Model file for the job. Use its own axes, mm. Coordinates: 2 decimals unless noted, no trailing zeros. Loops run counter-clockwise (first coordinate to the right, second up) from the corner with the lowest first, then second, coordinate; pieces in that order, holes last. Notation, with made-up numbers: (-27.75, 61) - (26.25, 61) arc R26 ccw to (26.25, 99) - close; hole circle Ø6 at (-31, -19). An arc over 180 degrees is marked (long way). Write each question's results on one line, items separated by ' | '. Start each with the question number.
```python
from build123d import *

# Parameters (mm, degrees)
EXTRUDE_1_DEPTH = 7
FILLET_1_R      = 10


with BuildPart() as part:
    # 草图1 → 凸台-拉伸1 (new body)
    with BuildSketch(Plane.XY):
        Polygon((-79.488423121, 60.813672833), (-61.488423121, 60.813672833), (-35.816291974, -24.186327167), (-51.816291974, -24.186327167), (-51.816291974, -40.186327167), (-16.816291974, -40.186327167), (-16.816291974, 60.813672833), (40.511576879, 60.813672833), (40.511576879, 40.813672833), (10.511576879, -55.186327167), (-79.488423121, -55.186327167), align=None)
    extrude(amount=EXTRUDE_1_DEPTH)

    # 圆角1
    fillet_1_edges = [part.edges().sort_by_distance(p)[0] for p in [
        (40.511576879, 40.813672833, 3.5),
    ]]
    fillet(fillet_1_edges, radius=FILLET_1_R)


solid = part.part
```
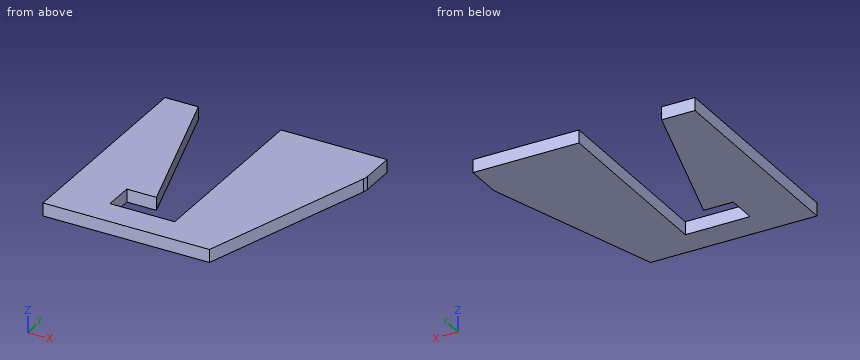
Q1. Pin check, flat tips, straight feed: pin 1 (4 mm diameter, centred on y = -10, z = 3.5, fed in from +X); pin 2 (3.5 mm diameter, centred on y = -29.5, z = 4.5, fed in from +X). Stop position of each tip, or through.
Q2. Drill centre lines: L1, parallel to X at y = -14.5, z = 4.75; L2, parallel to X at y = 15, z = 4.75; L3, parallel to Y at x = -25, z = 4.25. Where is each one in solid material? Low to high. Write a range as from..to.
Q3. Cut at A-A (x = -39). List the corners of the cut face in (y, z), and give its area (3 significant figures).
Q4. Cut at B-B (y = -18). List the corners of the cut face in (x, z).
Q5. Cut at D-D (x = 17.5). List the corners of the cut face in (y, z).
Q6. Cut at C-C (z = 1.5). List the corners of the cut face in (x, y).
Check result:
1) pin 1: x = 25.26 | pin 2: x = 19.09
2) L1: -79.49..-38.74, -16.82..23.23 | L2: -79.49..-47.65, -16.82..32.44 | L3: -55.19..-40.19
3) outline: (-55.19, 0) - (-40.19, 0) - (-40.19, 7) - (-55.19, 7) - close; (-24.19, 0) - (-13.65, 0) - (-13.65, 7) - (-24.19, 7) - close | area: 179 mm²
4) outline: (-79.49, 0) - (-37.68, 0) - (-37.68, 7) - (-79.49, 7) - close; (-16.82, 0) - (22.13, 0) - (22.13, 7) - (-16.82, 7) - close
5) outline: (-32.82, 0) - (60.81, 0) - (60.81, 7) - (-32.82, 7) - close
6) outline: (-79.49, -55.19) - (10.51, -55.19) - (40.06, 39.36) arc R10 ccw to (40.51, 42.34) - (40.51, 60.81) - (-16.82, 60.81) - (-16.82, -40.19) - (-51.82, -40.19) - (-51.82, -24.19) - (-35.82, -24.19) - (-61.49, 60.81) - (-79.49, 60.81) - close
